Could you check a few things on this model? Use its own coordinates, in mm. Face numbers are marked on the shaded views. A direction names the side the tool comes from. Coordinates: 2 decimals unless noted, no trailing zeros. Order: outer loops, then holes, each group sorted by start corner. A loop starts at its lowest first (then second) coordinate and runs counter-clockwise, first axis right, second up.
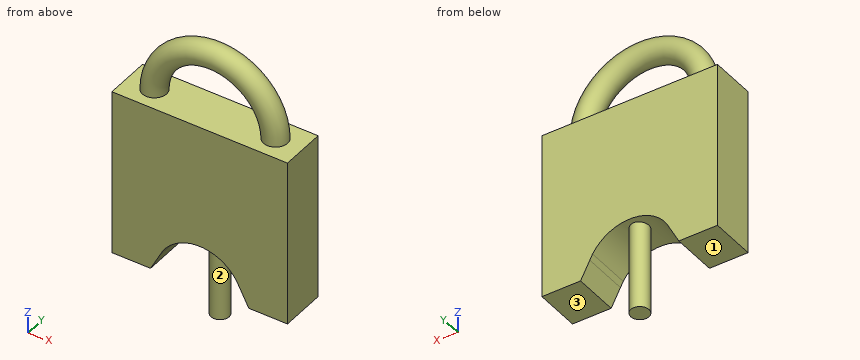
```python
from build123d import *

# Parameters (mm, degrees)
SKETCH1_R           = 1.5
BOSS_EXTRUDE1_DEPTH = 20
BOSS_EXTRUDE2_START = 15
BOSS_EXTRUDE2_DEPTH = 15
SWEEP1_PROFILE_R    = 2
BOSS_EXTRUDE3_DEPTH = 7.5
CHAMFER1_START      = -6
CHAMFER1_DEPTH      = 9
CHAMFER1_START_2    = -5
CHAMFER1_2_DEPTH    = 7.5


with BuildPart() as part:
    # Sketch1 → Boss-Extrude1 (new body)
    with BuildSketch(Plane.XY):
        Circle(SKETCH1_R)
    extrude(amount=-BOSS_EXTRUDE1_DEPTH)

    # Sketch1<3> → Boss-Extrude2 (add)
    with BuildSketch(Plane.XY.offset(BOSS_EXTRUDE2_START)):
        with BuildLine():
            Line((0, 1.5), (0, 2.5))
            Line((0, 2.5), (-14.5, 2.5))
            Line((-14.5, 2.5), (-14.5, -5))
            Line((-14.5, -5), (0, -5))
            Line((0, -5), (0, -1.5))
            ThreePointArc((0, -1.5), (-1.5, 0), (0, 1.5))
        make_face()
        with BuildLine():
            ThreePointArc((1.5, 0), (1.060660172, 1.060660172), (0, 1.5))
            Line((0, 1.5), (0, -1.5))
            ThreePointArc((0, -1.5), (1.060660172, -1.060660172), (1.5, 0))
        make_face()
        with BuildLine():
            Line((0, -1.5), (0, 1.5))
            ThreePointArc((0, 1.5), (-1.5, 0), (0, -1.5))
        make_face()
        with BuildLine():
            Line((14.5, 2.5), (0, 2.5))
            Line((0, 2.5), (0, 1.5))
            ThreePointArc((0, 1.5), (1.060660172, 1.060660172), (1.5, 0))
            ThreePointArc((1.5, 0), (1.060660172, -1.060660172), (0, -1.5))
            Line((0, -1.5), (0, -5))
            Line((0, -5), (14.5, -5))
            Line((14.5, -5), (14.5, 2.5))
        make_face()
    extrude(amount=-BOSS_EXTRUDE2_DEPTH)

    # Sweep1: sweep along a path in Sketch2
    with BuildLine(Plane(origin=(0, -1.25, 0), x_dir=(1, 0, 0), z_dir=(0, 1, 0))) as sweep1_path:
        ThreePointArc((-10, -15), (0, -25), (10, -15))
    # Sweep1 profile (on start of the path) → Sweep1 (sweep)
    with BuildSketch(Plane(origin=(-10, -1.25, 15), x_dir=(1, 0, 0), z_dir=(0, 0, 1))):
        Circle(SWEEP1_PROFILE_R)
    sweep(path=sweep1_path.line)

    # Sketch15 → Boss-Extrude3 (add)
    with BuildSketch(Plane(origin=(0, 2.5, 0), x_dir=(1, 0, 0), z_dir=(0, 1, 0))):
        with BuildLine():
            ThreePointArc((-7.2, 12.61), (0, 5.41), (7.2, 12.61))
            Line((7.2, 12.61), (14.5, 12.61))
            Line((14.5, 12.61), (14.5, 0))
            Line((14.5, 0), (-14.5, 0))
            Line((-14.5, 0), (-14.5, 12.61))
            Line((-14.5, 12.61), (-7.2, 12.61))
        make_face()
    extrude(amount=-BOSS_EXTRUDE3_DEPTH)

    # Chamfer1: read off the stored shape, not the designer's step
    # Chamfer1 outline → Chamfer1 (cut)
    with BuildSketch(Plane(origin=(0, 0, 0), x_dir=(1, 0, 0), z_dir=(0, 1, 0)).offset(CHAMFER1_START)):
        with BuildLine():
            ThreePointArc((7.2, 12.61), (7.04514475, 11.12476081), (6.587240153, 9.7034097))
            Line((6.587240153, 9.7034097), (8.114814982, 12.61))
            Line((8.114814982, 12.61), (7.2, 12.61))
        make_face()
        with BuildLine():
            Line((-8.114814982, 12.61), (-6.587240153, 9.7034097))
            ThreePointArc((-6.587240153, 9.7034097), (-7.04514475, 11.12476081), (-7.2, 12.61))
            Line((-7.2, 12.61), (-8.114814982, 12.61))
        make_face()
    extrude(amount=CHAMFER1_DEPTH, mode=Mode.SUBTRACT)

    # Chamfer1 2 outline → Chamfer1 2 (add)
    with BuildSketch(Plane(origin=(0, 0, 0), x_dir=(1, 0, 0), z_dir=(0, 1, 0)).offset(CHAMFER1_START_2)):
        with BuildLine():
            ThreePointArc((-6.587240153, 9.7034097), (-6.373406906, 9.260420263), (-6.129825647, 8.83306506))
            Line((-6.129825647, 8.83306506), (-6.587240153, 9.7034097))
        make_face()
        with BuildLine():
            Line((6.587240153, 9.7034097), (6.129825647, 8.83306506))
            ThreePointArc((6.129825647, 8.83306506), (6.373406906, 9.260420263), (6.587240153, 9.7034097))
        make_face()
    extrude(amount=CHAMFER1_2_DEPTH)


solid = part.part
```
Item 1: Suppose I cut it at A-A (x = 0). List the corners of the cut face in (y, z) for me.
Item 2: Suppose I cut it at D-D (y = -2.5). List the corners of the cut face in (x, z) for me, and give its area (3 significant figures).
Item 3: I need wall thicknesses on line 1 (X direction, y = -3.5, z = -6); line 2 (Z direction, x = -4.75, y = -1.5); line 3 (Z direction, x = -1.25, y = -0.75). Which ranges of each line are inside material? Lowest first, please.
Item 4: For pin 1 Ø3 at (x, y) = (-0.5, 1.5) entering from +Z, with a flat end and sliding along its axis, tell me the tip position at first contact or that it passes through.
Item 5: Which directions (+Z, -Z, +X, -X, +Y, -Y) give clear straight access to the entire face, cutting with the end or side of a thin tool? Please do the marked faces 1, 2 and 3.
Item 6: Suppose I cut it at B-B (y = -0.5). List the corners of the cut face in (x, z) for me.
Item 7: Suppose I cut it at C-C (z = -13.5). List the corners of the cut face in (x, y) for me, and give its area (3 significant figures).
Geometry results:
1. outline: (-5, -5.41) - (-1.5, -5.41) - (-1.5, -20) - (1.5, -20) - (1.5, -5.41) - (2.5, -5.41) - (2.5, 15) - (-5, 15) - close; circle Ø4 at (-1.25, 25)
2. outline: (-14.5, -12.61) - (-8.11, -12.61) - (-6.13, -8.83) arc R7.2 cw to (6.13, -8.83) - (8.11, -12.61) - (14.5, -12.61) - (14.5, 15) - (11.56, 15) arc R11.56 ccw to (-11.56, 15) - (-14.5, 15) - close; hole (-8.44, 15) - (8.44, 15) arc R8.44 ccw to start
2. area: 815 mm2
3. line 1: x = -14.5 to -2.85, 2.85 to 14.5
3. line 2: z = -7.2 to 15, 21.46 to 26
3. line 3: z = -20 to 15, 22.97 to 26.87
4. pin 1: stops at z = 26.55
5. face 1: -Z, -X, +Y, -Y
5. face 2: -Z
5. face 3: -Z, +X, +Y, -Y
6. outline: (-14.5, -12.61) - (-8.11, -12.61) - (-6.13, -8.83) arc R7.2 cw to (-1.41, -5.55) - (-1.41, -20) - (1.41, -20) - (1.41, -5.55) arc R7.2 cw to (6.13, -8.83) - (8.11, -12.61) - (14.5, -12.61) - (14.5, 15) - (11.85, 15) arc R11.85 ccw to (-11.85, 15) - (-14.5, 15) - close; hole (-8.15, 15) - (8.15, 15) arc R8.15 ccw to start
7. outline: circle Ø3 at (0, 0)
7. area: 7.07 mm2
